Work out the finished part from the listing and answer in its coordinate system (mm). Give positions to 0.01 mm unless a question says otherwise; leave off trailing zeros. Write each loop counter-clockwise with the first axis right and the second up, starting at its lowest first coordinate (ties: lowest second). Pieces come first, ordered by that corner, then holes.
1) Find section B-B (y = 0.8). Count the separate pieces of the cut face and the enclosed holes in it, plus the area to 3 significant figures.
2) Determine the mould class of faces 1 (the face through (-0.325, 1.479, 36.464)), 2 (the face through (8, 3, 8)), 3 (the face through (-8.67, 1.48, 39.05)), 4 (the face through (33.8, 1.5, 0.9)) for opening direction X: pulls with the +X half, pulls with the -X half, needs draft (parallel to the pull), parting line crosses it, or undercut.
3) Find section D-D (x = 35). Determine the outline of the cut face in (y, z).
4) Straight lines are drawn through the part: probe 1 along Z at (x, y) = (0, 1.65); probe 2 along Z at (x, y) = (-5.5, 0.4). For each, find the intervals that lie inside material, in ascending order.
5) Find section C-C (x = 0). Determine the outline of the cut face in (y, z).
6) Given pin 1 Ø1.5 at (x, y) = (22, 2.5) entering from -Z; pin 2 Ø1 at (x, y) = (27.5, 2.5) entering from -Z; pin 3 Ø2.5 at (x, z) = (10, 10) entering from -Y; pin 4 Ø1.5 at (x, y) = (-15, 1) entering from -Z, each flat-ended and moving along its own axis, determine where each tip first touches the part or whether it passes through.
7) Find section A-A (z = 0). Determine the outline of the cut face in (x, y), plus the area to 3 significant figures.
```python
from build123d import *

# Parameters (mm, degrees)
SKETCH1_R           = 40
SKETCH1_R_2         = 1.5
BOSS_EXTRUDE1_DEPTH = 3
SKETCH2_R           = 1.5
CUT_EXTRUDE1_DEPTH  = 3
SKETCH3_R           = 10
CUT_EXTRUDE2_DEPTH  = 10


with BuildPart() as part:
    # Sketch1 → Boss-Extrude1 (new body)
    with BuildSketch(Plane(origin=(0, 0, 0), x_dir=(1, 0, 0), z_dir=(0, 1, 0))):
        Circle(SKETCH1_R)
        with Locations((0, 35)):
            Circle(SKETCH1_R_2, mode=Mode.SUBTRACT)
        with Locations((35, 0)):
            Circle(SKETCH1_R_2, mode=Mode.SUBTRACT)
        with Locations((0, -35)):
            Circle(SKETCH1_R_2, mode=Mode.SUBTRACT)
        with Locations((-35, 0)):
            Circle(SKETCH1_R_2, mode=Mode.SUBTRACT)
    extrude(amount=BOSS_EXTRUDE1_DEPTH)

    # Sketch2 → Cut-Extrude1 (cut)
    with BuildSketch(Plane(origin=(0, 3, 0), x_dir=(1, 0, 0), z_dir=(0, 1, 0))):
        with Locations((10, 10)):
            Circle(SKETCH2_R)
        with Locations((-10, 10)):
            Circle(SKETCH2_R)
        with Locations((-10, -10)):
            Circle(SKETCH2_R)
        with Locations((10, -10)):
            Circle(SKETCH2_R)
    extrude(amount=-CUT_EXTRUDE1_DEPTH, mode=Mode.SUBTRACT)

    # Sketch3 → Cut-Extrude2 (cut)
    with BuildSketch(Plane(origin=(0, 3, 0), x_dir=(1, 0, 0), z_dir=(0, 1, 0))):
        Circle(SKETCH3_R)
    extrude(amount=-CUT_EXTRUDE2_DEPTH, mode=Mode.SUBTRACT)


solid = part.part
```
Results:
1. separate pieces: 1
1. enclosed holes: 9
1. area: 4,660 mm2
2. face 1: undercut
2. face 2: needs draft
2. face 3: parting line crosses it
2. face 4: undercut
3. outline: (0, -19.36) - (3, -19.36) - (3, -1.5) - (0, -1.5) - close; (0, 1.5) - (3, 1.5) - (3, 19.36) - (0, 19.36) - close
4. probe 1: z = -40 to -36.5, -33.5 to -10, 10 to 33.5, 36.5 to 40
4. probe 2: z = -39.62 to -8.35, 8.35 to 39.62
5. outline: (0, -40) - (3, -40) - (3, -36.5) - (0, -36.5) - close; (0, -33.5) - (3, -33.5) - (3, -10) - (0, -10) - close; (0, 10) - (3, 10) - (3, 33.5) - (0, 33.5) - close; (0, 36.5) - (3, 36.5) - (3, 40) - (0, 40) - close
6. pin 1: stops at z = -33.89
6. pin 2: stops at z = -29.51
6. pin 3: passes through
6. pin 4: stops at z = -37.38
7. outline: (-40, 0) - (-36.5, 0) - (-36.5, 3) - (-40, 3) - close; (-33.5, 0) - (-10, 0) - (-10, 3) - (-33.5, 3) - close; (10, 0) - (33.5, 0) - (33.5, 3) - (10, 3) - close; (36.5, 0) - (40, 0) - (40, 3) - (36.5, 3) - close
7. area: 162 mm2
